Verification items for this drawing (mm, ordinates from the low corner). A direction names the side the tool comes from. Round coordinates to 2 decimals unless told otherwise and drop trailing zeros. Loops run counter-clockwise (first coordinate to the right, second up) from the corner with the lowest first, then second, coordinate; pieces in that order, holes last. Notation, with made-up numbers: M 30,-17 L 57,-17 A12 ccw 57,3 Z; hole C 59,19.25 d7. An arc over 180 degrees is marked long. Write item = value, one per line.
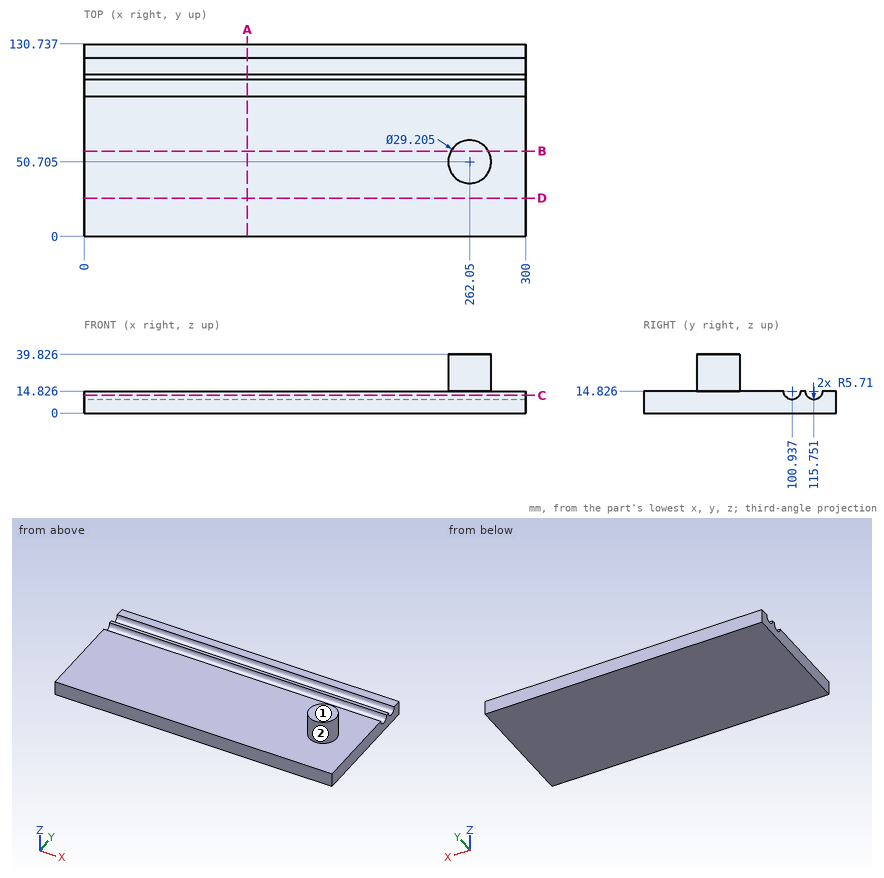
(1) Sectioned sample at D-D on y = 26. Record the cut outline in (x, z) (1 decimal), then the cut area to 3 significant figures.
Result set:
outline = M 0,0 L 300,0 L 300,14.8 L 0,14.8 Z
area = 4,450 mm2
(2) Material ranges on line 1 along Z through (x, y) = (220, 94.5) (1 decimal); line 2 along Y through (x, z) = (254, 25); line 3 along Z through (x, y) = (283.5, 96.5), recorded low to high. Write a range as from..to.
Result set:
line_1 = 0..14.8
line_2 = 38.52..62.89
line_3 = 0..11.23
(3) Sectioned sample at C-C on z = 12. Record the cut outline in (x, y) (1 decimal), then the cut area to 3 significant figures.
Result set:
outline = M 0,0 L 300,0 L 300,96 L 0,96 Z; M 0,105.9 L 300,105.9 L 300,110.8 L 0,110.8 Z; M 0,120.7 L 300,120.7 L 300,130.7 L 0,130.7 Z
area = 33,300 mm2
(4) Tool access check on the marked faces 1 and 2. Record the directions out of +Z, -Z, +X, -X, +Y, -Y that give a thin tool (end or side, any length) a straight path to the whole face; none if there is none.
Result set:
face_1 = +Z, +X, -X, +Y, -Y
face_2 = +Z
(5) Sectioned sample at B-B on y = 58. Record the cut outline in (x, z) (1 decimal).
Result set:
outline = M 0,0 L 300,0 L 300,14.8 L 274.7,14.8 L 274.7,39.8 L 249.4,39.8 L 249.4,14.8 L 0,14.8 Z
(6) Depth check by flat-ended pin: pin 1 Ø2 at (x, y) = (91, 69.5) entering from -Z; pin 2 Ø12 at (x, y) = (39.5, 13.5) entering from +Z. Enter the tip coordinate at first touch or a pass-through.
Result set:
pin_1 = 0
pin_2 = 14.83
(7) Sectioned sample at A-A on x = 111. Record the cut outline in (y, z) (1 decimal).
Result set:
outline = M 0,0 L 130.7,0 L 130.7,14.8 L 121.5,14.8 A5.7 cw 110,14.8 L 106.6,14.8 A5.7 cw 95.2,14.8 L 0,14.8 Z
